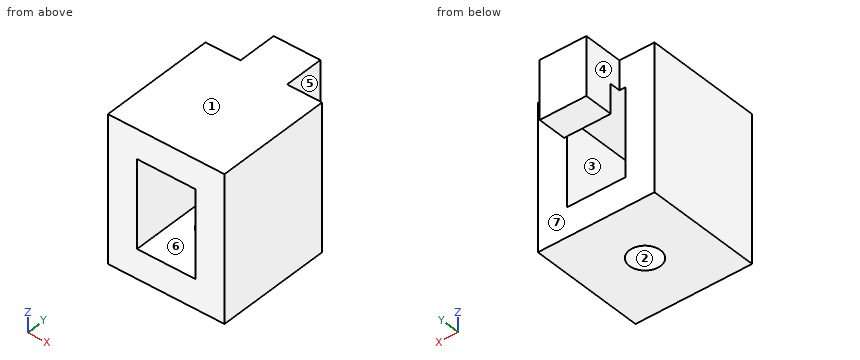
```python
from build123d import *

# Parameters (mm, degrees)
SKETCH1_W                  = 20
SKETCH1_H                  = 20
BOSS_EXTRUDE1_DEPTH        = 5
F_4_0_209_DIAMETER_HOLE1_D = 5.3086
BOSS_EXTRUDE5_START        = 5
SKETCH1_5_W                = 5
SKETCH1_5_H                = 20
BOSS_EXTRUDE5_DEPTH        = 15
BOSS_EXTRUDE6_START        = 20
SKETCH1_6_W                = 5
SKETCH1_6_H                = 20
BOSS_EXTRUDE6_DEPTH        = 5
BOSS_EXTRUDE7_START        = 25
SKETCH1_7_W                = 8
SKETCH1_7_H                = 1.8
BOSS_EXTRUDE7_DEPTH        = 5
BOSS_EXTRUDE8_START        = 25
SKETCH1_8_W                = 8
SKETCH1_8_H                = 5
BOSS_EXTRUDE8_DEPTH        = 10


with BuildPart() as part:
    # Sketch1 → Boss-Extrude1 (new body)
    with BuildSketch(Plane.XY):
        Rectangle(SKETCH1_W, SKETCH1_H)
    extrude(amount=BOSS_EXTRUDE1_DEPTH)

    # #4 (0.209) Diameter Hole1 (through all)
    with Locations(Plane.XY.offset(5)):
        with Locations((0, 0)):
            Hole(F_4_0_209_DIAMETER_HOLE1_D / 2)

    # Sketch1<5> → Boss-Extrude5 (add)
    with BuildSketch(Plane.XY.offset(BOSS_EXTRUDE5_START)):
        with Locations((-7.5, 0)):
            Rectangle(SKETCH1_5_W, SKETCH1_5_H)
        with Locations((7.5, 0)):
            Rectangle(SKETCH1_5_W, SKETCH1_5_H)
    extrude(amount=BOSS_EXTRUDE5_DEPTH)

    # Sketch1<6> → Boss-Extrude6 (add)
    with BuildSketch(Plane.XY.offset(BOSS_EXTRUDE6_START)):
        with Locations((-7.5, 0)):
            Rectangle(SKETCH1_6_W, SKETCH1_6_H)
        Polygon((4, 10), (-4, 10), (-5, 10), (-5, -10), (5, -10), (5, 10), align=None)
        with Locations((7.5, 0)):
            Rectangle(SKETCH1_6_W, SKETCH1_6_H)
    extrude(amount=BOSS_EXTRUDE6_DEPTH)

    # Sketch1<7> → Boss-Extrude7 (add)
    with BuildSketch(Plane.XY.offset(BOSS_EXTRUDE7_START)):
        with Locations((0, 10.9)):
            Rectangle(SKETCH1_7_W, SKETCH1_7_H)
    extrude(amount=-BOSS_EXTRUDE7_DEPTH)

    # Sketch1<8> → Boss-Extrude8 (add)
    with BuildSketch(Plane.XY.offset(BOSS_EXTRUDE8_START)):
        with Locations((0, 14.3)):
            Rectangle(SKETCH1_8_W, SKETCH1_8_H)
    extrude(amount=-BOSS_EXTRUDE8_DEPTH)


solid = part.part
```
Can you work these out from the model? Positions are in its coordinate system, mm. Face numbers are marked on the shaded views. A direction names the side the tool comes from. Give positions to 0.01 mm unless a question says otherwise; leave off trailing zeros. Loops run counter-clockwise (first coordinate to the right, second up) from the corner with the lowest first, then second, coordinate; pieces in that order, holes last. Notation, with made-up numbers: M -10,26.25 L 18,26.25 A29 cw 18,59.25 Z; hole C -21,18 d3. An arc over 180 degrees is marked long. Answer in a Markdown table with one row per item.
1. Suppose I cut it at B-B on y = 7.75. Write out the boundary of the cut face in (x, z).
Taken from the geometry:
| item | result |
|---|---|
| outline | M -10,0 L 10,0 L 10,25 L -10,25 Z; hole M -5,5 L 5,5 L 5,20 L -5,20 Z |
2. Suppose I cut it at C-C on x = 0. Write out the boundary of the cut face in (y, z), plus the area to 3 significant figures.
Taken from the geometry:
| item | result |
|---|---|
| outline | M -10,0 L -2.65,0 L -2.65,5 L -10,5 Z; M -10,20 L 11.8,20 L 11.8,15 L 16.8,15 L 16.8,25 L -10,25 Z; M 2.65,0 L 10,0 L 10,5 L 2.65,5 Z |
| area | 232 mm² |
3. Thinking about a two-plate mould opening in Z: for the marked faces 1, 2 and 3, which applies, released by +Z, released by -Z, zero draft, split by the parting line, or undercut?
Taken from the geometry:
| item | result |
|---|---|
| face 1 | released by +Z |
| face 2 | zero draft |
| face 3 | undercut |
4. For pin 1 Ø8 at (x, y) = (0, 3.5) entering from -Z; pin 2 Ø2 at (y, z) = (12, 19) entering from -X; pin 3 Ø5.5 at (y, z) = (15, 17.5) entering from +X; pin 4 Ø1.5 at (x, z) = (1, 17.5) entering from -Y, each with a flat end and sliding along its axis, tell me the tip position at first contact or that it passes through.
Taken from the geometry:
| item | result |
|---|---|
| pin 1 | stops at z = 0 |
| pin 2 | stops at x = -4 |
| pin 3 | stops at x = 4 |
| pin 4 | stops at y = 11.8 |
5. If I drill on line 1 along X through (y, z) = (6, 19.75); line 2 along Z through (x, y) = (4.75, 4); line 3 along Y through (x, z) = (0, 1.15), over which ranges is the centre line in solid material (lowest first)?
Taken from the geometry:
| item | result |
|---|---|
| line 1 | x = -10 to -5, 5 to 10 |
| line 2 | z = 0 to 5, 20 to 25 |
| line 3 | y = -10 to -2.65, 2.65 to 10 |
6. Suppose I cut it at A-A on z = 18. Write out the boundary of the cut face in (x, y), plus the area to 3 significant figures.
Taken from the geometry:
| item | result |
|---|---|
| outline | M -10,-10 L -5,-10 L -5,10 L -10,10 Z; M -4,11.8 L 4,11.8 L 4,16.8 L -4,16.8 Z; M 5,-10 L 10,-10 L 10,10 L 5,10 Z |
| area | 240 mm² |
7. Which directions (+Z, -Z, +X, -X, +Y, -Y) give clear straight access to the entire face, cutting with the end or side of a thin tool? Please do the marked faces 4, 5, 6 and 7.
Taken from the geometry:
| item | result |
|---|---|
| face 4 | +Z, -Z, -X, +Y |
| face 5 | +Z, -Z, +X, +Y |
| face 6 | +Y, -Y |
| face 7 | -Z, +Y |
8. Suppose I cut it at D-D on z = 7.5. Write out the boundary of the cut face in (x, y), plus the area to 3 significant figures.
Taken from the geometry:
| item | result |
|---|---|
| outline | M -10,-10 L -5,-10 L -5,10 L -10,10 Z; M 5,-10 L 10,-10 L 10,10 L 5,10 Z |
| area | 200 mm² |
